```python
from build123d import *

# Parameters (mm, degrees)
F1_DEPTH      = 45
F1_DEPTH_BACK = 45
F2_W          = 67
F2_H          = 5
F3_DEPTH      = 40
F3_DEPTH_BACK = 40
F5_R          = 1.5
F6_DEPTH      = 30
F8_DEPTH      = 8
F9_R          = 4
F10_T1_DEPTH  = 20
F10_T3_DEPTH  = 16.1803398875


# Not quite as in the source:
# - a fillet or chamfer that OpenCascade refuses, or shapes differently, is made with other operations: its cross-section is extruded or revolved along the edge and cut away or added


with BuildPart() as f1:
    # F0 (on Front) → F1 (new body, two sides)
    with BuildSketch(Plane.XZ) as f1_sk:
        Polygon((0, 50), (0, 0), (70, 0), (70, 10), (10, 10), (10, 50), align=None)
    extrude(amount=F1_DEPTH)
    extrude(f1_sk.sketch, amount=-F1_DEPTH_BACK)

    # F2 (on Front) → F3 (join, two sides)
    with BuildSketch(Plane.XZ) as f3_sk:
        with Locations((32.5, 39.3734816462)):
            Rectangle(F2_W, F2_H)
    extrude(amount=-F3_DEPTH)
    extrude(f3_sk.sketch, amount=F3_DEPTH_BACK)

    # F5 (on offset) → F6 (cut)
    with BuildSketch(Plane.XY.offset(55)):
        with Locations((7, -35)):
            Circle(F5_R)
        with Locations((7, 35)):
            Circle(F5_R)
    extrude(amount=-F6_DEPTH, mode=Mode.SUBTRACT)

    # F7 (on face) → F8 (cut)
    with BuildSketch(Plane.XY.offset(10)):
        with BuildLine():
            ThreePointArc((68.5, 40.5), (67.6213203436, 42.6213203436), (65.5, 43.5))
            Line((65.5, 43.5), (13, 43.5))
            ThreePointArc((13, 43.5), (10.8786796564, 42.6213203436), (10, 40.5))
            Line((10, 40.5), (10, -40.5))
            ThreePointArc((10, -40.5), (10.8786796564, -42.6213203436), (13, -43.5))
            Line((13, -43.5), (65.5, -43.5))
            ThreePointArc((65.5, -43.5), (67.6213203436, -42.6213203436), (68.5, -40.5))
            Line((68.5, -40.5), (68.5, 40.5))
        make_face()
    extrude(amount=-F8_DEPTH, mode=Mode.SUBTRACT)

    # F9
    f9_edges = [f1.edges().sort_by_distance(p)[0] for p in [
        (70, -45, 5),
        (70, 45, 5),
        (0, -45, 25),
        (0, 45, 25),
        (10, -45, 30),
        (10, 45, 30),
    ]]
    fillet(f9_edges, radius=F9_R)

    # F10: fillet of radius 3 on 4 edges, made by hand

    # F10_s2 → F10_t1 (cut)
    with BuildSketch(Plane.XY.offset(29.3734816462)):
        with BuildLine():
            ThreePointArc((63, -40), (65.1213203436, -39.1213203436), (66, -37))
            Line((66, -37), (66, -40))
            Line((66, -40), (63, -40))
        make_face()
        with BuildLine():
            ThreePointArc((63, 40), (65.1213203436, 39.1213203436), (66, 37))
            Line((66, 37), (66, 40))
            Line((66, 40), (63, 40))
        make_face()
    extrude(amount=F10_T1_DEPTH, mode=Mode.SUBTRACT)

    # F10_s4 → F10_t3 (cut)
    with BuildSketch(Plane.XY.offset(31.2833117024)):
        with BuildLine():
            ThreePointArc((0, 40), (-0.7386127875, 38.9886768939), (-1, 37.7639320225))
            Line((-1, 37.7639320225), (-1, 40))
            Line((-1, 40), (0, 40))
        make_face()
        with BuildLine():
            ThreePointArc((0, -40), (-0.7386127875, -38.9886768939), (-1, -37.7639320225))
            Line((-1, -37.7639320225), (-1, -40))
            Line((-1, -40), (0, -40))
        make_face()
    extrude(amount=F10_T3_DEPTH, mode=Mode.SUBTRACT)


solid = f1.part
```
Verification items for the finished model (mm, model axes). A direction names the side the tool comes from. Round coordinates to 2 decimals unless told otherwise and drop trailing zeros. Write each loop counter-clockwise with the first axis right and the second up, starting at its lowest first coordinate (ties: lowest second). Pieces come first, ordered by that corner, then holes.
1. Gauge pin test, flat ends, axial feed: P1, Ø2, axis at x = 29.5, y = -16.5, coming from the +Z side; P2, Ø2.5, axis at x = 7, y = 35, coming from the +Z side; P3, Ø4, axis at y = 2.5, z = 40.5, coming from the +X side. Record the tip position at first contact, or that the pin passes through.
2. Draft check along Y on faces 1 (the flat face through (40, 43.5, 6)), 2 (the cylindrical face through (6.675, 33.536, 37.675)), 3 (the cylindrical face through (8.797, 43.859, 30.28)), 4 (the cylindrical face through (8.797, -43.859, 30.28)). Enter one of: +Y half, -Y half, draft (parallel to the pull), parting line (faces both ways), or undercut.
3. Section check D-D on y = 1.5. Enter the section's corners in (x, z), plus the area to 3 significant figures.
4. Section check C-C on y = 35. Enter the section's corners in (x, z).
5. Section check A-A on x = 28. Enter the section's corners in (y, z).
6. Section check B-B on z = 11.5. Enter the section's corners in (x, y).
7. Scan lines: L1, parallel to Z at x = 50.5, y = 33.5; L2, parallel to X at y = 35, z = 7.5; L3, parallel to Y at x = 7, z = 42. Record each from-to range of solid material in increasing order.
8. Access from +Z, -Z, +X, -X, +Y, -Y to the whole of each face (thin tool, end or side, straight path). Record for faces 5 (the cylindrical face through (65.1, 39.14, 39.34)), 6 (the cylindrical face through (6.675, -36.464, 37.675)), 7 (the flat face through (38, -1, 41.873)).
Answer:
1. P1: stops at z = 41.87
1. P2: stops at z = 25
1. P3: stops at x = 66
2. face 1: undercut
2. face 2: undercut
2. face 3: +Y half
2. face 4: -Y half
3. outline: (-1, 36.87) - (0, 36.87) - (0, 0) - (70, 0) - (70, 10) - (68.5, 10) - (68.5, 2) - (10, 2) - (10, 36.87) - (66, 36.87) - (66, 41.87) - (10, 41.87) - (10, 50) - (0, 50) - (0, 41.87) - (-1, 41.87) - close
3. area: 917 mm2
4. outline: (-1, 36.87) - (0, 36.87) - (0, 0) - (70, 0) - (70, 10) - (68.5, 10) - (68.5, 2) - (10, 2) - (10, 36.87) - (66, 36.87) - (66, 41.87) - (10, 41.87) - (10, 50) - (8.5, 50) - (8.5, 25) - (5.5, 25) - (5.5, 50) - (0, 50) - (0, 41.87) - (-1, 41.87) - close
5. outline: (-45, 0) - (45, 0) - (45, 10) - (43.5, 10) - (43.5, 2) - (-43.5, 2) - (-43.5, 10) - (-45, 10) - close; (-40, 36.87) - (40, 36.87) - (40, 41.87) - (-40, 41.87) - close
6. outline: (0, -41) arc R4 ccw to (4, -45) - (6, -45) arc R4 ccw to (10, -41) - (10, 41) arc R4 ccw to (6, 45) - (4, 45) arc R4 ccw to (0, 41) - close
7. L1: z = 0 to 2, 36.87 to 41.87
7. L2: x = 0 to 10, 68.5 to 70
7. L3: y = -44.87 to -36.5, -33.5 to 33.5, 36.5 to 44.87
8. face 5: +Z, +X, +Y
8. face 6: +Z
8. face 7: +Z, +X, +Y, -Y
